Part model, mm, in its own coordinate system. A direction names the side the tool comes from. Round coordinates to 2 decimals unless told otherwise and drop trailing zeros. Loops run counter-clockwise (first coordinate to the right, second up) from the corner with the lowest first, then second, coordinate; pieces in that order, holes last.
(1) Cut at C-C on x = -20. List the corners of the cut face in (y, z), then the cut area to 4 significant figures.
(2) Cut at B-B on y = -35. List the corners of the cut face in (x, z), then the cut area to 4 significant figures.
(3) Mould opens along X. For faces 4 (the face through (-21.03, 38.52, 9.86)), 5 (the face through (35, 10, -5)), 6 (the face through (0, 1, 0)), 7 (the face through (30, 25, 10)) say: +X half, -X half, draft (parallel to the pull), parting line (faces both ways), or undercut.
(4) Probe probe 1 along X at (y, z) = (26, 3.5); probe 2 along Z at (x, y) = (-28, -10); probe 3 along Y at (x, z) = (28.5, 12). List the from-to ranges inside material, lowest first.
(5) Flat gauge pins, fed straight in: pin 1 (4 mm diameter, centred on x = -3, z = 8.5, fed in from -Y); pin 2 (12 mm diameter, centred on y = 14, z = 10, fed in from -X); pin 3 (5 mm diameter, centred on x = 28, z = 12, fed in from -Y); pin 4 (8 mm diameter, centred on x = 3, z = 11.5, fed in from -Y). Where does each tip first touch, or does it go through?
(6) Cut at D-D on y = -20. List the corners of the cut face in (x, z), then the cut area to 3 significant figures.
(7) Tool access for faces 1 (the face through (1.34, -32.89, 12.32)), 2 (the face through (-10, 49, 10)), 3 (the face through (-30, 25, 10)): list every direction of +Z, -Z, +X, -X, +Y, -Y with a clear straight run to the whole face (end or side of a thin tool).
(8) Cut at A-A on z = 3. List the corners of the cut face in (x, y).
from build123d import *

# Parameters (mm, degrees)
F0_W     = 70
F0_H     = 100
F1_DEPTH = 15
F3_DEPTH = 20
F4_R     = 2.5
F5_DEPTH = 25


with BuildPart() as f1:
    # F0 (on Top) → F1 (new body)
    with BuildSketch(Plane.XY):
        Rectangle(F0_W, F0_H)
    extrude(amount=-F1_DEPTH)

    # F2 (on face) → F3 (join)
    with BuildSketch(Plane.XY):
        with BuildLine():
            Line((-10, 47.912878), (-10, 50))
            Line((-10, 50), (-35, 50))
            Line((-35, 50), (-35, 25))
            Line((-35, 25), (-25, 25))
            ThreePointArc((-25, 25), (-20.916501, 38.693064), (-10, 47.912878))
        make_face()
        with BuildLine():
            ThreePointArc((10, 47.912878), (20.916501, 38.693064), (25, 25))
            Line((25, 25), (35, 25))
            Line((35, 25), (35, 50))
            Line((35, 50), (10, 50))
            Line((10, 50), (10, 47.912878))
        make_face()
    extrude(amount=F3_DEPTH)

    # F4 (on face) → F5 (join)
    with BuildSketch(Plane.XY):
        with Locations((-20, -20)):
            Circle(F4_R)
        with Locations((0, -35)):
            Circle(F4_R)
        with Locations((20, -20)):
            Circle(F4_R)
    extrude(amount=F5_DEPTH)


solid = f1.part
Final values:
1. outline: (-50, -15) - (50, -15) - (50, 20) - (40, 20) - (40, 0) - (-17.5, 0) - (-17.5, 25) - (-22.5, 25) - (-22.5, 0) - (-50, 0) - close
1. area: 1,825 mm2
2. outline: (-35, -15) - (35, -15) - (35, 0) - (2.5, 0) - (2.5, 25) - (-2.5, 25) - (-2.5, 0) - (-35, 0) - close
2. area: 1,175 mm2
3. face 4: undercut
3. face 5: +X half
3. face 6: undercut
3. face 7: draft
4. probe 1: x = -35 to -24.98, 24.98 to 35
4. probe 2: z = -15 to 0
4. probe 3: y = 25 to 50
5. pin 1: stops at y = -37.29
5. pin 2: passes through
5. pin 3: stops at y = 25
5. pin 4: stops at y = -37.5
6. outline: (-35, -15) - (35, -15) - (35, 0) - (22.5, 0) - (22.5, 25) - (17.5, 25) - (17.5, 0) - (-17.5, 0) - (-17.5, 25) - (-22.5, 25) - (-22.5, 0) - (-35, 0) - close
6. area: 1,300 mm2
7. face 1: +Z
7. face 2: +Z, +Y, -Y
7. face 3: +Z, +X, -X, -Y
8. outline: (-35, 25) - (-25, 25) arc R25 cw to (-10, 47.91) - (-10, 50) - (-35, 50) - close; circle Ø5 at (-20, -20); circle Ø5 at (0, -35); (10, 47.91) arc R25 cw to (25, 25) - (35, 25) - (35, 50) - (10, 50) - close; circle Ø5 at (20, -20)
